For this review, take the finished solid that the model builds, in its own axes (mm). Face numbers are marked on the shaded views. A direction names the side the tool comes from. Coordinates: 2 decimals unless noted, no trailing zeros. Loops run counter-clockwise (first coordinate to the right, second up) from the corner with the lowest first, then second, coordinate; pieces in that order, holes last. Notation, with made-up numbers: M 65.25,39 L 88.25,39 A18 ccw 88.25,47 Z; hole C -22.5,43.5 d5. An arc over 180 degrees is marked long. Write item = value, one per line.
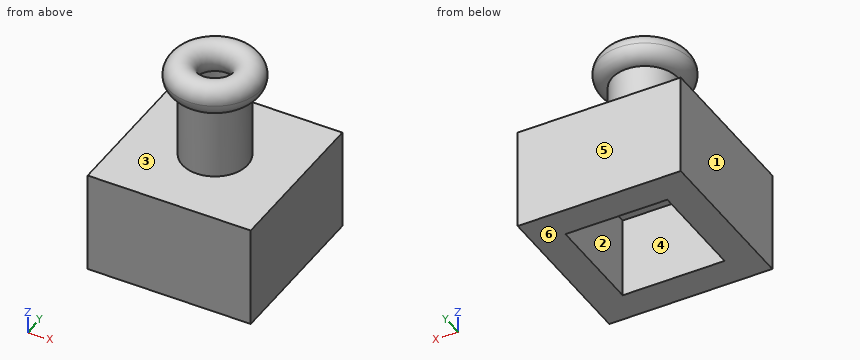
from build123d import *

# Parameters (mm, degrees)
BOX001_W          = 10
BOX001_H          = 10
BOX001_DEPTH      = 8
BOX_W             = 16
BOX_H             = 16
BOX_DEPTH         = 10
TORUS_R           = 1.5
CYLINDER_R        = 2.5
CYLINDER_DEPTH    = 9
CYLINDER001_R     = 3.2
CYLINDER001_DEPTH = 9


with BuildPart() as cube001:
    # Box001 → Box001 (new body)
    with BuildSketch(Plane(origin=(-5, -5, 0), x_dir=(1, 0, 0), z_dir=(0, 0, 1))):
        with Locations((5, 5)):
            Rectangle(BOX001_W, BOX001_H)
    extrude(amount=BOX001_DEPTH)


with BuildPart() as cube:
    # Box → Box (new body)
    with BuildSketch(Plane(origin=(-8, -8, 0), x_dir=(1, 0, 0), z_dir=(0, 0, 1))):
        with Locations((8, 8)):
            Rectangle(BOX_W, BOX_H)
    extrude(amount=BOX_DEPTH)


with BuildPart() as torus:
    # Torus → Torus (revolve)
    with BuildSketch(Plane(origin=(0, 0, 18.5), x_dir=(1, 0, 0), z_dir=(0, -1, 0))):
        with Locations((3, 0)):
            Circle(TORUS_R)
    revolve(axis=Axis((0, 0, 18.5), (0, 0, 1)))


with BuildPart() as cylinder:
    # Cylinder → Cylinder (new body)
    with BuildSketch(Plane.XY.offset(10)):
        Circle(CYLINDER_R)
    extrude(amount=CYLINDER_DEPTH)


with BuildPart() as cut001:
    # Cylinder001 → Cylinder001 (new body)
    with BuildSketch(Plane.XY.offset(10)):
        Circle(CYLINDER001_R)
    extrude(amount=CYLINDER001_DEPTH)

    # Cut: cut Cylinder
    add(cylinder.part, mode=Mode.SUBTRACT)

    # Fusion: union Cube, Torus
    add(cube.part)
    add(torus.part)

    # Cut001: cut Cube001
    add(cube001.part, mode=Mode.SUBTRACT)


solid = cut001.part
Q1. Draft analysis for pull direction Y (two halves, no side actions). For the marked faces 4, 5 and 6, state which applies: +Y half, -Y half, draft (parallel to the pull), parting line (faces both ways), or undercut.
Solved:
face_4 = undercut
face_5 = +Y half
face_6 = draft
Q2. For pin 1 Ø4.5 at (x, y) = (0, 0) entering from +Z; pin 2 Ø1.5 at (x, y) = (1, 1) entering from +Z; pin 3 Ø2 at (y, z) = (-1.5, 15.5) entering from -X, all flat-tipped, find the tip position at first contact; note any pin that passes through.
Solved:
pin_1 = 19.8
pin_2 = 19.75
pin_3 = -3.16
Q3. For line 1 along Y through (x, z) = (-4, 4.25); line 2 along Y through (x, z) = (0, 13.5); line 3 along Z through (x, y) = (-4.25, -6.75), list the stretches that pass through material, from the lowest coordinate up.
Solved:
line_1 = -8 to -5, 5 to 8
line_2 = -3.2 to -2.5, 2.5 to 3.2
line_3 = 0 to 10
Q4. Add section A-A (z = 4.5). Write out the cut boundary in (x, y), and give its area (3 significant figures).
Solved:
outline = M -8,-8 L 8,-8 L 8,8 L -8,8 Z; hole M -5,-5 L 5,-5 L 5,5 L -5,5 Z
area = 156 mm²
Q5. Machinability: for the marked faces 1, 2 and 3, which of the approach directions +Z, -Z, +X, -X, +Y, -Y give a long, thin tool a straight path to every point of the face, cutting with its end or side? Answer none if there is none.
Solved:
face_1 = +Z, -Z, -X, +Y, -Y
face_2 = -Z
face_3 = none
Q6. Add section D-D (z = 16). Write out the cut boundary in (x, y).
Solved:
outline = C 0,0 d6.4; hole C 0,0 d5
Q7. Add section B-B (y = 0). Write out the cut boundary in (x, z), and give its area (3 significant figures).
Solved:
outline = M -8,0 L -5,0 L -5,8 L 5,8 L 5,0 L 8,0 L 8,10 L 3.2,10 L 3.2,17.01 A1.5 ccw long 2.5,17.09 L 2.5,10 L -2.5,10 L -2.5,17.09 A1.5 ccw long -3.2,17.01 L -3.2,10 L -8,10 Z
area = 104 mm²
